from build123d import *

# Parameters (mm, degrees)
EXTRUDE_1_DEPTH     = 3
CUT_EXTRUDE_1_DEPTH = 5
EXTRUDE_2_DEPTH     = 5
SKETCH_4_R          = 1.25
SKETCH_4_R_2        = 1.5
SKETCH_4_W          = 3
SKETCH_4_H          = 15
CUT_EXTRUDE_2_DEPTH = 5
FILLET_1_R          = 3
FILLET_2_R          = 5
SKETCH_5_R          = 10
SKETCH_5_R_2        = 1.5
CUT_EXTRUDE_3_DEPTH = 10
FILLET_3_R          = 1


with BuildPart() as part:
    # 草图1 → 凸台-拉伸1 (new body)
    with BuildSketch(Plane(origin=(0, 0, 0), x_dir=(1, 0, 0), z_dir=(0, 1, 0))):
        with BuildLine():
            Line((0, 0), (0, -135))
            ThreePointArc((0, -135), (113.857845185, -72.535447127), (122.35155125, 57.053465335))
            Line((122.35155125, 57.053465335), (0, 0))
        make_face()
    extrude(amount=EXTRUDE_1_DEPTH)

    # 草图2 → 切除-拉伸1 (cut)
    with BuildSketch(Plane(origin=(0, 3, 0), x_dir=(1, 0, 0), z_dir=(0, 1, 0))):
        with BuildLine():
            Line((0, 0), (104.225395509, 48.6011001))
            ThreePointArc((104.225395509, 48.6011001), (107.568320743, -40.670091868), (46, -105.399240984))
            Line((46, -105.399240984), (54, -123.729543764))
            ThreePointArc((54, -123.729543764), (27.581801898, -132.152352246), (0, -135))
            Line((0, -135), (0, 0))
        make_face()
    extrude(amount=-CUT_EXTRUDE_1_DEPTH, mode=Mode.SUBTRACT)

    # 草图3 → 凸台-拉伸2 (add)
    with BuildSketch(Plane(origin=(0, 3, 0), x_dir=(1, 0, 0), z_dir=(0, 1, 0))):
        with BuildLine():
            Line((46, -105.399240984), (54, -123.729543764))
            ThreePointArc((54, -123.729543764), (88.040639509, -102.341808636), (114.273799591, -71.878360632))
            ThreePointArc((114.273799591, -71.878360632), (95.730838943, -107.385901313), (83.09704134, -145.399240984))
            Line((83.09704134, -145.399240984), (18.09704134, -145.399240984))
            ThreePointArc((18.09704134, -145.399240984), (8.158015649, -136.501859828), (15.905249936, -125.642394647))
            ThreePointArc((15.905249936, -125.642394647), (32.852844555, -118.345804202), (46, -105.399240984))
        make_face()
    extrude(amount=-EXTRUDE_2_DEPTH)

    # 草图4 → 切除-拉伸2 (cut)
    with BuildSketch(Plane(origin=(0, 3, 0), x_dir=(1, 0, 0), z_dir=(0, 1, 0))):
        with Locations((126, -8)):
            Circle(SKETCH_4_R)
        with Locations((126, -17)):
            Circle(SKETCH_4_R)
        with Locations((18.09704134, -135.399240984)):
            Circle(SKETCH_4_R_2)
        with Locations((53.261619346, -113.641470943)):
            Circle(SKETCH_4_R)
        with Locations((61.682428963, -110.465000355)):
            Circle(SKETCH_4_R)
        with Locations((121.091047045, 39.915013787)):
            Circle(SKETCH_4_R_2)
        with Locations((126.614572621, 15)):
            Circle(SKETCH_4_R_2)
        Polygon((59.901130208, -97.242785157), (60.959953737, -100.049721696), (46.925271043, -105.343839343), (45.866447513, -102.536902804), align=None)
        with Locations((114.5, -12.5)):
            Rectangle(SKETCH_4_W, SKETCH_4_H)
    extrude(amount=-CUT_EXTRUDE_2_DEPTH, mode=Mode.SUBTRACT)

    # 圆角1
    fillet_1_edges = [part.edges().sort_by_distance(p)[0] for p in [
        (104.225395509, 1.5, -48.6011001),
        (122.35155125, 1.5, -57.053465335),
    ]]
    fillet(fillet_1_edges, radius=FILLET_1_R)

    # 圆角2
    fillet_2_edges = [part.edges().sort_by_distance(p)[0] for p in [
        (83.09704134, 0.5, 145.399240984),
    ]]
    fillet(fillet_2_edges, radius=FILLET_2_R)

    # 草图5 → 切除-拉伸3 (cut)
    with BuildSketch(Plane(origin=(0, 3, 0), x_dir=(1, 0, 0), z_dir=(0, 1, 0))):
        with Locations((47.633497714, -128.622545035)):
            Circle(SKETCH_5_R)
        with Locations((78.536756787, -138.249693791)):
            Circle(SKETCH_5_R_2)
        with Locations((74.091279988, -130.424239426)):
            Circle(SKETCH_5_R_2)
        with BuildLine():
            Line((68.829172362, -98.298245315), (84.88931258, -121.234502555))
            ThreePointArc((84.88931258, -121.234502555), (93.343637557, -99.289475714), (103.822616306, -78.23595301))
            Line((103.822616306, -78.23595301), (95.836261206, -72.217802778))
            ThreePointArc((95.836261206, -72.217802778), (83.359004455, -86.320776041), (68.829172362, -98.298245315))
        make_face()
        with BuildLine():
            Line((101.765771539, -63.590311708), (110.2462525, -68.88950435))
            ThreePointArc((110.2462525, -68.88950435), (119.665630949, -50.795046704), (126.138444416, -31.449846428))
            Line((126.138444416, -31.449846428), (116.435487153, -29.030627472))
            ThreePointArc((116.435487153, -29.030627472), (110.460582414, -46.887735419), (101.765771539, -63.590311708))
        make_face()
    extrude(amount=-CUT_EXTRUDE_3_DEPTH, mode=Mode.SUBTRACT)

    # 圆角3
    fillet_3_edges = [part.edges().sort_by_distance(p)[0] for p in [
        (101.765771539, 1.5, 63.590311708),
        (116.435487153, 1.5, 29.030627472),
        (126.138444416, 1.5, 31.449846428),
        (110.2462525, 1.5, 68.88950435),
        (68.829172362, 1.5, 98.298245315),
        (95.836261206, 1.5, 72.217802778),
        (103.822616306, 1.5, 78.23595301),
        (84.88931258, 0.5, 121.234502555),
    ]]
    fillet(fillet_3_edges, radius=FILLET_3_R)


solid = part.part
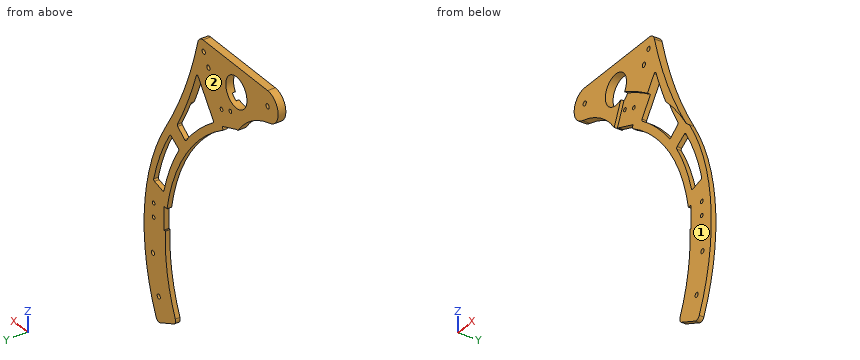
Check sheet for the modelled part. Datum: model origin and axes. Units: mm. Face numbers are marked on the shaded views. A direction names the side the tool comes from. Round coordinates to 2 decimals unless told otherwise and drop trailing zeros. Order: outer loops, then holes, each group sorted by start corner. A loop starts at its lowest first (then second) coordinate and runs counter-clockwise, first axis right, second up.
Q1. Cross-section at C-C, the plane x = 29. Enter the section's corners in (y, z).
Filled sheet:
outline: (-2, 120.69) - (3, 120.69) - (3, 145.4) - (-2, 145.4) - close
Q2. Set-up check for the marked faces 1 and 2: record each of +Z, -Z, +X, -X, +Y, -Y from which the full face is reachable in a straight line by a thin tool's end or side.
Filled sheet:
face 1: -Z, -Y
face 2: +Z, -Z, +X, -X, +Y
Q3. Cross-section at B-B, the plane y = -0.8. Enter the section's corners in (x, z), plus the area to 3 significant figures.
Filled sheet:
outline: (15.91, 125.64) arc R50 cw to (46, 105.4) - (52.27, 119.76) arc R10 cw (long way) to (55.84, 122.91) arc R135 cw to (77.43, 110.59) - (83.75, 119.61) arc R1 cw to (85.52, 119.36) arc R250 ccw to (94.74, 96.17) arc R135 cw to (114.27, 71.88) arc R250 cw to (84.04, 141.67) arc R5 ccw to (79.21, 145.4) - (18.1, 145.4) arc R10 ccw to start; hole circle Ø3 at (18.1, 135.4); hole circle Ø3 at (74.09, 130.42); hole circle Ø3 at (78.54, 138.25)
area: 1,940 mm2
Q4. Cross-section at D-D, the plane z = 22. Enter the section's corners in (x, y).
Filled sheet:
outline: (112.88, 0) - (133.2, 0) - (133.2, 3) - (112.88, 3) - close
Q5. Scan lines: L1, parallel to X at y = 1.35, z = 17; L2, parallel to Y at x = 116, z = 67.5; L3, parallel to X at y = 1.8, z = 67. Record each from-to range of solid material in increasing order.
Filled sheet:
L1: x = 116 to 124.75, 127.25 to 133.93
L2: y = 0 to 3
L3: x = 93.47 to 107.22, 111.4 to 117.2
Q6. Cross-section at A-A, the plane z = 45. Enter the section's corners in (x, y).
Filled sheet:
outline: (105.83, 0) - (111.24, 0) - (111.24, 3) - (105.83, 3) - close; (121.96, 0) - (127.28, 0) - (127.28, 3) - (121.96, 3) - close
Q7. Depth check by flat-ended pin: P1, Ø2.5, axis at x = 74.09, z = 130.42, coming from the -Y side; P2, Ø3, axis at y = 0.5, z = 61, coming from the -X side; P3, Ø0.9, axis at x = 115.5, y = 1.5, coming from the +Z side; P4, Ø1.4, axis at x = 115, y = 1.5, coming from the -Z side. Enter the tip coordinate at first touch or a pass-through.
Filled sheet:
P1: passes through
P2: stops at x = 96.53
P3: stops at z = 70.63
P4: stops at z = -53.95
